Source: CAD feature listing. Evaluate the final solid. Frame: model axes, mm. A direction names the side the tool comes from. Give positions to 0.01 mm unless a question says otherwise; leave off trailing zeros. Order: outer loops, then holes, each group sorted by start corner. A loop starts at its lowest first (then second) coordinate and runs counter-clockwise, first axis right, second up. Notation, with made-up numbers: M 83,8.25 L 126,8.25 A20 ccw 126,27.25 Z; hole C 67.25,-9 d2. An arc over 180 degrees is marked long. Use CSV: the item, a comma, the result in double quotes. Start each with the question number.
Item 1: Ray query, probe 1 along Z at (x, y) = (-19.5, 51); probe 2 along X at (y, z) = (-17.5, 39.5); probe 3 along Y at (x, z) = (4, 92.5). Return the intervals inside material, ascending. Write a range as from..to.
Item 2: Pull-direction query (X, two-part tool) for faces 1 (the face through (26, 21, 98)), 2 (the face through (20, 25, 72)), 3 (the face through (-5, -25, 72)); classes: +X half, -X half, draft (parallel to the pull), parting line (faces both ways), or undercut.
Item 3: Section query C-C on x = -3. Return loops of the section in (y, z), and give its area (3 significant figures).
Item 4: Section query D-D on z = 37. Return loops of the section in (x, y).
Item 5: Access query for faces 4 (the face through (25, 20, 72)), 5 (the face through (-1, 60, 37)), 6 (the face through (5, -25, 72)), 7 (the face through (-30, 25, 75)). Directions: +Z, -Z, +X, -X, +Y, -Y. A direction counts if a zero-diameter tool reaches every point of the face in a straight line with its end or side. Return the directions, or none.
Item 6: First-contact query: pin 1 (11 mm diameter, centred on y = 24.5, z = 77.5, fed in from -X); pin 2 (5 mm diameter, centred on x = -23.5, z = 79.5, fed in from +Y); pin 3 (5 mm diameter, centred on x = -0.5, z = 62.5, fed in from +Y); pin 4 (3 mm diameter, centred on x = 29, y = -27, fed in from -Z). Flat tips, straight axial feed; report the tip coordinate or a pass-through.
Item 7: Section query A-A on z = 77. Return loops of the section in (x, y), and give its area (3 significant figures).
Item 8: Section query B-B on y = -4.5. Return loops of the section in (x, z).
from build123d import *

# Parameters (mm, degrees)
F0_W     = 150
F0_H     = 150
F1_DEPTH = 25
F2_W     = 120
F2_H     = 120
F3_DEPTH = 25
F4_W     = 10
F4_H     = 10
F5_DEPTH = 50
F6_R     = 4.99999


# Not quite as in the source:
# - a fillet or chamfer is up to 0.001 mm smaller than in the source, because OpenCascade refuses the exact size


with BuildPart() as f1:
    # F0 (on Top) → F1 (new body)
    with BuildSketch(Plane.XY):
        Rectangle(F0_W, F0_H)
    extrude(amount=F1_DEPTH)

    # F2 (on face) → F3 (join)
    with BuildSketch(Plane.XY.offset(25)):
        Rectangle(F2_W, F2_H)
    extrude(amount=F3_DEPTH)

    # F4 (on face) → F5 (join)
    with BuildSketch(Plane.XY.offset(50)):
        with Locations((0, -25)):
            Rectangle(F4_W, F4_H)
        with Locations((-25, 25)):
            Rectangle(F4_W, F4_H)
        with Locations((25, 25)):
            Rectangle(F4_W, F4_H)
    extrude(amount=F5_DEPTH)

    # F6 (radius 5 in the source; OpenCascade refuses exactly that, so slightly less here)
    f6_edges = [f1.edges().sort_by_distance(p)[0] for p in [
        (-25, 20, 100),
        (-20, 25, 100),
        (25, 20, 100),
        (20, 25, 100),
        (-5, -25, 100),
        (0, -20, 100),
        (5, -25, 100),
    ]]
    fillet(f6_edges, radius=F6_R)


solid = f1.part
Verdict:
1,probe 1,"0..50"
1,probe 2,"-60..60"
1,probe 3,"-30..-20"
2,face 1,"draft"
2,face 2,"undercut"
2,face 3,"-X half"
3,outline,"M -75,0 L 75,0 L 75,25 L 60,25 L 60,50 L -20,50 L -20,95 A5 ccw -22,99 L -30,99 L -30,50 L -60,50 L -60,25 L -75,25 Z"
3,area,"7,240 mm2"
4,outline,"M -60,-60 L 60,-60 L 60,60 L -60,60 Z"
5,face 4,"+Z, +X, -X, -Y"
5,face 5,"+Z, +X, -X, +Y"
5,face 6,"+Z, +X, +Y, -Y"
5,face 7,"+Z, -X, +Y, -Y"
6,pin 1,"x = -30"
6,pin 2,"y = 30"
6,pin 3,"y = -20"
6,pin 4,"z = 0"
7,outline,"M -30,20 L -20,20 L -20,30 L -30,30 Z; M -5,-30 L 5,-30 L 5,-20 L -5,-20 Z; M 20,20 L 30,20 L 30,30 L 20,30 Z"
7,area,"300 mm2"
8,outline,"M -75,0 L 75,0 L 75,25 L 60,25 L 60,50 L -60,50 L -60,25 L -75,25 Z"
